Geometry: see drawing. Coordinates: mm, zero at the bounding-box minimum. A direction names the side the tool comes from. Round coordinates to 2 decimals unless told otherwise and drop trailing zeros. Order: outer loops, then holes, each group sorted by start corner. A loop starts at its lowest first (then second) coordinate and runs counter-clockwise, first axis right, second up. Notation, with made-up numbers: (72.5, 71) -> (131.5, 71) arc R23 ccw to (131.5, 109) -> close; hole circle Ø7 at (0.25, 63). An arc over 180 degrees is marked (long way). Use a Markdown table: item, result.
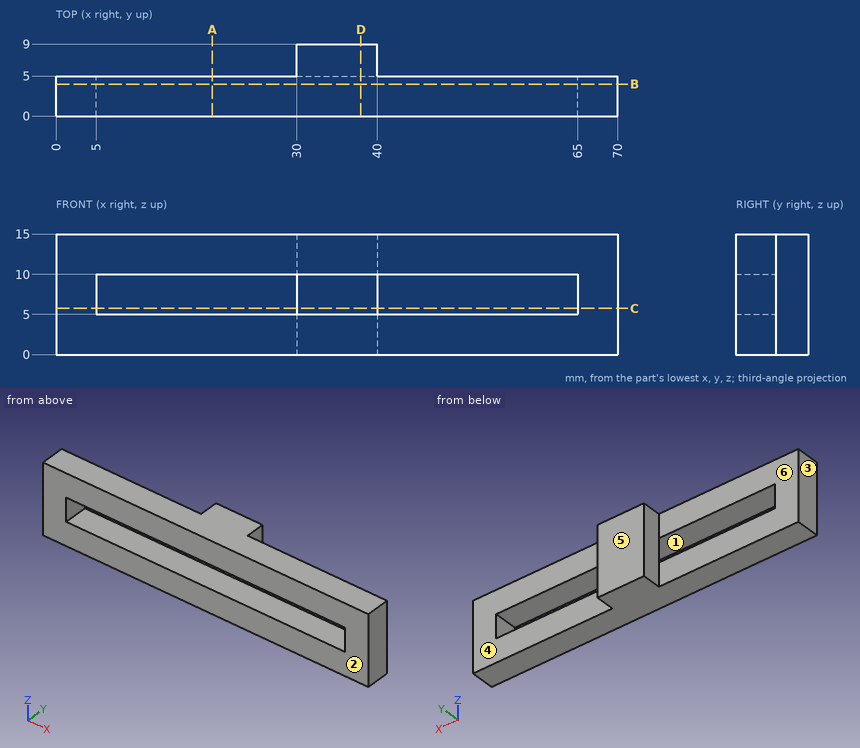
1) Cut plane D-D on x = 38. Return loops of the section in (y, z), and give its area (3 significant figures).
Answer key:
| item | result |
|---|---|
| outline | (0, 0) -> (9, 0) -> (9, 15) -> (0, 15) -> (0, 10) -> (5, 10) -> (5, 5) -> (0, 5) -> close |
| area | 110 mm^2 |
2) Cut plane C-C on z = 5.75. Return loops of the section in (x, y), and give its area (3 significant figures).
Answer key:
| item | result |
|---|---|
| outline | (0, 0) -> (5, 0) -> (5, 5) -> (0, 5) -> close; (30, 5) -> (40, 5) -> (40, 9) -> (30, 9) -> close; (65, 0) -> (70, 0) -> (70, 5) -> (65, 5) -> close |
| area | 90.0 mm^2 |
3) Draft query along X for the marked faces 1, 2 and 3. Return one class per face: released by +X, released by -X, zero draft, split by the parting line, or undercut.
Answer key:
| item | result |
|---|---|
| face 1 | undercut |
| face 2 | zero draft |
| face 3 | released by -X |
4) Ray query, probe 1 along Z at (x, y) = (9, 4.75); probe 2 along X at (y, z) = (2.25, 5.75); probe 3 along Y at (x, z) = (33, 9). Return the intervals inside material, ascending.
Answer key:
| item | result |
|---|---|
| probe 1 | z = 0 to 5, 10 to 15 |
| probe 2 | x = 0 to 5, 65 to 70 |
| probe 3 | y = 5 to 9 |
5) Contact query for flat-ended pins moving along their axis: P1, Ø1.2, axis at y = 7.5, z = 7.5, coming from the +X side; P2, Ø1.5, axis at y = 6.5, z = 3.5, coming from the -X side. Output: stop coordinate, or through.
Answer key:
| item | result |
|---|---|
| P1 | stops at x = 40 |
| P2 | stops at x = 30 |
6) Set-up query: the marked faces 4, 5 and 6. Return all of +Z, -Z, +X, -X, +Y, -Y with unobstructed straight access to the full face (end or side cutting, diameter ignored); none if empty.
Answer key:
| item | result |
|---|---|
| face 4 | +Z, -Z, +X, +Y |
| face 5 | +Z, -Z, +X, -X, +Y |
| face 6 | +Z, -Z, -X, +Y |
7) Cut plane A-A on x = 19.5. Return loops of the section in (y, z).
Answer key:
| item | result |
|---|---|
| outline | (0, 0) -> (5, 0) -> (5, 5) -> (0, 5) -> close; (0, 10) -> (5, 10) -> (5, 15) -> (0, 15) -> close |
8) Cut plane B-B on y = 4. Return loops of the section in (x, z).
Answer key:
| item | result |
|---|---|
| outline | (0, 0) -> (70, 0) -> (70, 15) -> (0, 15) -> close; hole (5, 5) -> (65, 5) -> (65, 10) -> (5, 10) -> close |
